Here's the drawing with two shaded views (mm, measured from the low corner). I have some questions. Give positions to 0.01 mm unless a question says otherwise; leave off trailing zeros. Write each loop counter-clockwise with the first axis right and the second up, starting at its lowest first coordinate (ties: lowest second). Pieces come first, ordered by that corner, then holes. Notation, with made-up numbers: (37.5, 74) -> (76.5, 74) arc R20 ccw to (76.5, 87) -> close; hole circle Ø9 at (52.5, -22). An arc over 180 degrees is marked (long way). One line per item, written item: value.
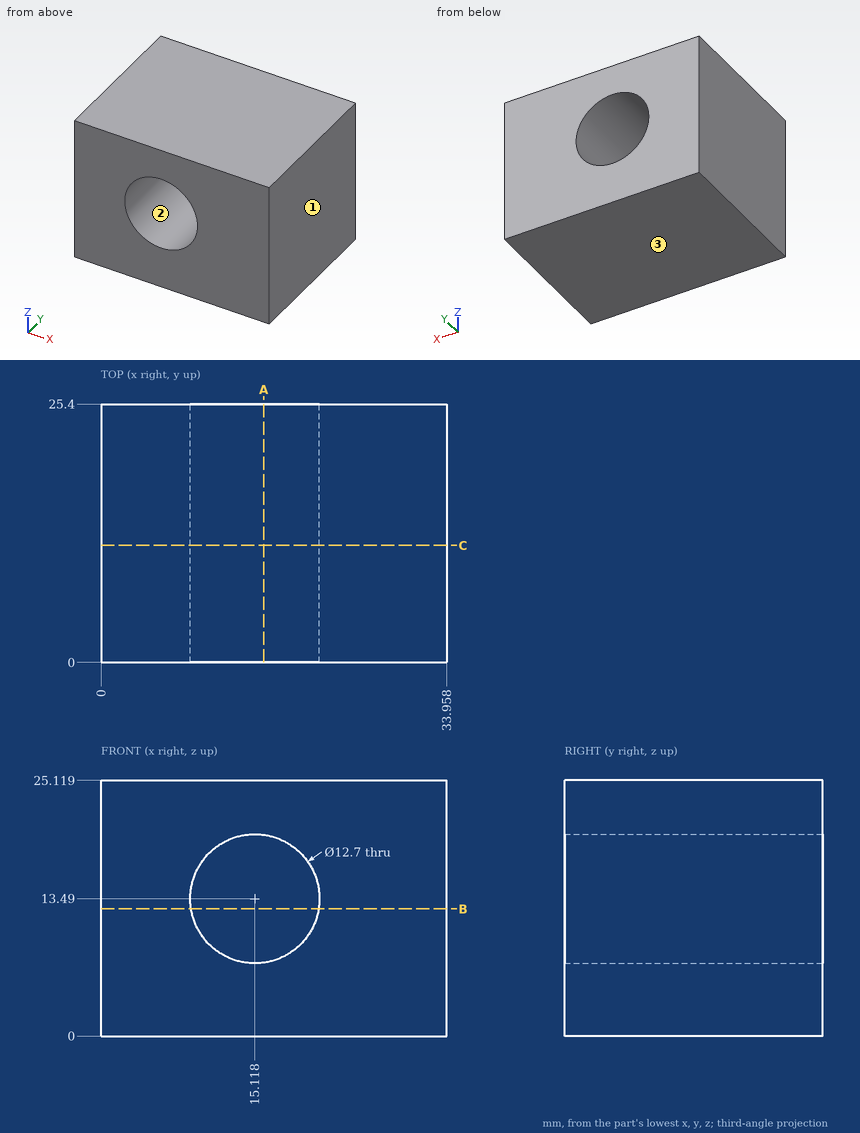
1) I need wall thicknesses on L1, parallel to X at y = 17, z = 13.25; L2, parallel to Z at x = 18, y = 24.5; L3, parallel to X at y = 3.25, z = 7.75 (1 decimal). Which ranges of each line are inside material? Lowest first, please.
Answer list:
L1: x = 0 to 8.77, 21.46 to 33.96
L2: z = 0 to 7.83, 19.15 to 25.12
L3: x = 0 to 12.4, 17.8 to 34
2) If we section it at C-C (y = 11.5): Write out the boundary of the cut face in (x, z), and give its area (3 significant figures).
Answer list:
outline: (0, 0) -> (33.96, 0) -> (33.96, 25.12) -> (0, 25.12) -> close; hole circle Ø12.7 at (15.12, 13.49)
area: 726 mm^2
3) We'd pull the mould along Z, two halves only. Please class the marked faces 1, 2 and 3: released by +Z, released by -Z, zero draft, split by the parting line, or undercut.
Answer list:
face 1: zero draft
face 2: undercut
face 3: released by -Z
4) Will this pin go through, and if not, where does the flat tip stop? pin 1 (7.5 mm diameter, centred on x = 15.12, z = 13.49, fed in from +Y).
Answer list:
pin 1: passes through
5) If we section it at A-A (x = 16): Write out the boundary of the cut face in (y, z).
Answer list:
outline: (0, 0) -> (25.4, 0) -> (25.4, 7.2) -> (0, 7.2) -> close; (0, 19.78) -> (25.4, 19.78) -> (25.4, 25.12) -> (0, 25.12) -> close
6) If we section it at B-B (z = 12.5): Write out the boundary of the cut face in (x, y) (1 decimal).
Answer list:
outline: (0, 0) -> (8.8, 0) -> (8.8, 25.4) -> (0, 25.4) -> close; (21.4, 0) -> (34, 0) -> (34, 25.4) -> (21.4, 25.4) -> close
